from build123d import *

# Parameters (mm, degrees)
SCHIZZO1_W                       = 500
SCHIZZO1_H                       = 300
ESTRUSIONE_ESTRUSIONE1_DEPTH     = 3
SCHIZZO2_W                       = 20
SCHIZZO2_H                       = 20
ESTRUSIONE_ESTRUSIONE2_DEPTH     = 1305
RIPETIZIONE_A_L1_COUNT           = 2
RIPETIZIONE_A_L1_PITCH           = 400
RIPETIZIONE_A_L2_COUNT           = 2
RIPETIZIONE_A_L2_PITCH           = 200
RIPETIZIONE_A_L2_COPY_1_SKETCH_W = 20
RIPETIZIONE_A_L2_COPY_1_SKETCH_H = 20
RIPETIZIONE_A_L2_COPY_1_DEPTH    = 1305


with BuildPart() as part:
    # Schizzo1 → Estrusione-Estrusione1 (new body)
    with BuildSketch(Plane.XY):
        Rectangle(SCHIZZO1_W, SCHIZZO1_H)
    extrude(amount=ESTRUSIONE_ESTRUSIONE1_DEPTH)

    # Schizzo2 → Estrusione-Estrusione2 (add)
    with BuildSketch(Plane.XY.offset(3)):
        with Locations((-200, 100)):
            Rectangle(SCHIZZO2_W, SCHIZZO2_H)
    estrusione_estrusione2 = extrude(amount=ESTRUSIONE_ESTRUSIONE2_DEPTH)

    # Ripetizione a L1: Estrusione-Estrusione2 ×2
    with Locations(*[(i * RIPETIZIONE_A_L1_PITCH, 0, 0) for i in range(1, RIPETIZIONE_A_L1_COUNT)]):
        add(estrusione_estrusione2)

    # Ripetizione a L2: Estrusione-Estrusione2 ×2
    with Locations(*[(0, -i * RIPETIZIONE_A_L2_PITCH, 0) for i in range(1, RIPETIZIONE_A_L2_COUNT)]):
        add(estrusione_estrusione2)

    # Ripetizione a L2 copy 1 sketch → Ripetizione a L2 copy 1 (add)
    with BuildSketch(Plane(origin=(400, -200, 3), x_dir=(1, 0, 0), z_dir=(0, 0, 1))):
        with Locations((-200, 100)):
            Rectangle(RIPETIZIONE_A_L2_COPY_1_SKETCH_W, RIPETIZIONE_A_L2_COPY_1_SKETCH_H)
    extrude(amount=RIPETIZIONE_A_L2_COPY_1_DEPTH)


solid = part.part
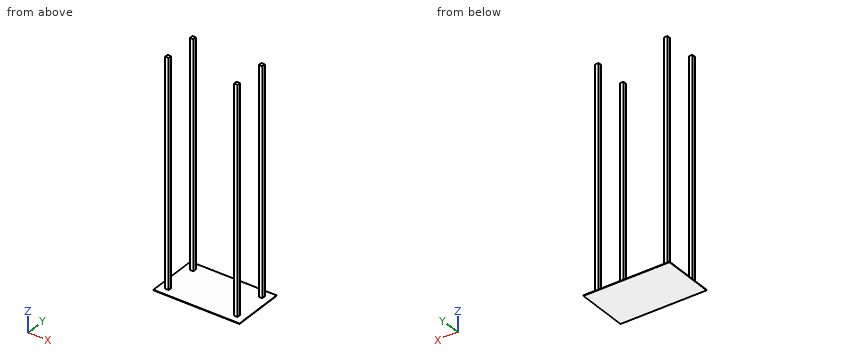
Check sheet for the modelled part. Datum: model origin and axes. Units: mm. Give positions to 0.01 mm unless a question says otherwise; leave off trailing zeros. Loops run counter-clockwise (first coordinate to the right, second up) from the corner with the lowest first, then second, coordinate; pieces in that order, holes last. Notation, with made-up numbers: M 7,-17.75 L 30,-17.75 A14 ccw 30,0.25 Z; hole C -39.75,43.5 d9. An arc over 180 degrees is marked long. Answer as a JSON object with one key per item and string values. Group by question number.
Q1. Go/stop test with flat-tipped pins: P1, Ø22, axis at y = -100.5, z = 859, coming from the -X side; P2, Ø6, axis at x = 198.5, z = 788, coming from the +Y side; P3, Ø22, axis at x = 201, z = 706.5, coming from the -Y side. Record where each tip stops, or that it passes through.
Q2. Cross-section at A-A on z = 465. Record the cut outline in (x, y).
Q3. Cross-section at B-B on x = 156.5. Record the cut outline in (y, z), then the cut area to 3 significant figures.
Q4. Material ranges on line 1 along Y through (x, z) = (-196, 803.5); line 2 along X through (y, z) = (109, 813.5); line 3 along Z through (x, y) = (126.5, 87.5), recorded low to high. Write a range as [from, to].
Q5. Cross-section at C-C on y = 122. Record the cut outline in (x, z).
Evaluation:
{
 "1": {"P1": "stops at x = -210", "P2": "stops at y = 110", "P3": "stops at y = -110"},
 "2": {"outline": "M -210,-110 L -190,-110 L -190,-90 L -210,-90 Z; M -210,90 L -190,90 L -190,110 L -210,110 Z; M 190,-110 L 210,-110 L 210,-90 L 190,-90 Z; M 190,90 L 210,90 L 210,110 L 190,110 Z"},
 "3": {"outline": "M -150,0 L 150,0 L 150,3 L -150,3 Z", "area": "900 mm2"},
 "4": {"line 1": "y = [-110, -90], [90, 110]", "line 2": "x = [-210, -190], [190, 210]", "line 3": "z = [0, 3]"},
 "5": {"outline": "M -250,0 L 250,0 L 250,3 L -250,3 Z"}
}
